Source: CAD feature listing. Evaluate the final solid. Frame: model axes, mm. A direction names the side the tool comes from. Give positions to 0.01 mm unless a question says otherwise; leave off trailing zeros. Order: outer loops, then holes, each group sorted by start corner. A loop starts at its lowest first (then second) coordinate and runs counter-clockwise, first axis right, second up.
1) Section D-D, the plane y = 74.5. Return loops of the section in (x, z) (3 decimals).
2) Section C-C, the plane z = 2.4. Give the number of separate pieces and of enclosed holes in the cut face, plus the area to 3 significant figures.
3) First-contact query: P1, Ø6.5, axis at x = 38.1, y = 12.7, coming from the +Z side (3 decimals); P2, Ø1.6, axis at y = 19.5, z = 2.5, coming from the +X side; P3, Ø1, axis at x = 298.5, z = 2.5, coming from the -Y side; P4, Ø1.6, axis at x = 217, z = 1, coming from the -Y side. Flat tips, straight axial feed; report the tip coordinate or a pass-through.
4) Access query for faces 4 (the face through (125.09, 1.81, 1.61)), 5 (the face through (105.885, 71.607, 1.61)). Directions: +Z, -Z, +X, -X, +Y, -Y. A direction counts if a zero-diameter tool reaches every point of the face in a straight line with its end or side. Return the directions, or none.
5) Draft query along X for faces 1 (the face through (138, 73, 0)), 2 (the face through (32.161, 71.607, 1.61)), 3 (the face through (20, 75.4, 1.6)). Return one class per face: released by +X, released by -X, zero draft, split by the parting line, or undercut.
6) Material intervals for line 1 (X direction, y = 35, z = 1.85); line 2 (X direction, y = 67, z = 1.9); line 3 (Y direction, x = 184, z = 2), sorted ascending.
7) Section A-A, the plane y = 95.5. Return loops of the section in (x, z) (3 decimals).
8) Section B-B, the plane x = 232.5. Return loops of the section in (y, z) (3 decimals), plus the area to 3 significant figures.
```python
from build123d import *

# Parameters (mm, degrees)
SKETCH1_R           = 2.54
SKETCH1_R_2         = 2.159
BOSS_EXTRUDE1_DEPTH = 3.175
FILLET1_R           = 6.35
CUT_EXTRUDE1_DEPTH  = 354.562731103
FILLET2_R           = 3.175
SKETCH3_R           = 2.54
CUT_EXTRUDE2_DEPTH  = 354.562731103
FILLET3_R           = 3.175


with BuildPart() as part:
    # Sketch1 → Boss-Extrude1 (new body)
    with BuildSketch(Plane.XY):
        with BuildLine():
            Line((40.64, 127), (0, 25.4))
            Line((0, 25.4), (0, 0))
            Line((0, 0), (127, 0))
            Line((127, 0), (127, 25.4))
            Line((127, 25.4), (152.4, 88.9))
            Line((152.4, 88.9), (278.011284287, 88.9))
            ThreePointArc((278.011284287, 88.9), (326.39, 107.95), (278.011284287, 127))
            Line((278.011284287, 127), (40.64, 127))
        make_face()
        with Locations((12.7, 12.7)):
            Circle(SKETCH1_R, mode=Mode.SUBTRACT)
        with Locations((38.1, 12.7)):
            Circle(SKETCH1_R, mode=Mode.SUBTRACT)
        with Locations((63.5, 12.7)):
            Circle(SKETCH1_R, mode=Mode.SUBTRACT)
        with Locations((88.9, 12.7)):
            Circle(SKETCH1_R, mode=Mode.SUBTRACT)
        with Locations((114.3, 12.7)):
            Circle(SKETCH1_R, mode=Mode.SUBTRACT)
        with Locations((286.54375, 128.572229928)):
            Circle(SKETCH1_R_2, mode=Mode.SUBTRACT)
        with Locations((310.35625, 128.572229928)):
            Circle(SKETCH1_R_2, mode=Mode.SUBTRACT)
        with Locations((310.35625, 87.327770072)):
            Circle(SKETCH1_R_2, mode=Mode.SUBTRACT)
        with Locations((286.54375, 87.327770072)):
            Circle(SKETCH1_R_2, mode=Mode.SUBTRACT)
        Polygon((302.409468146, 101.092), (294.490531854, 101.092), (290.531063708, 107.95), (294.490531854, 114.808), (302.409468146, 114.808), (306.368936292, 107.95), align=None, mode=Mode.SUBTRACT)
        with Locations((274.6375, 107.95)):
            Circle(SKETCH1_R_2, mode=Mode.SUBTRACT)
        with Locations((322.2625, 107.95)):
            Circle(SKETCH1_R_2, mode=Mode.SUBTRACT)
    extrude(amount=BOSS_EXTRUDE1_DEPTH)

    # Fillet1
    fillet1_edges = [part.edges().sort_by_distance(p)[0] for p in [
        (278.011284287, 88.9, 1.5875),
        (152.4, 88.9, 1.5875),
        (127, 25.4, 1.5875),
        (127, 0, 1.5875),
        (0, 0, 1.5875),
        (0, 25.4, 1.5875),
        (40.64, 127, 1.5875),
        (278.011284287, 127, 1.5875),
    ]]
    fillet(fillet1_edges, radius=FILLET1_R)

    # Sketch2 → Cut-Extrude1 (cut, through all)
    with BuildSketch(Plane.XY.offset(3.175)):
        Polygon((49.23831861, 114.3), (13.67831861, 25.4), (39.597669611, 25.4), (75.157669611, 114.3), align=None)
        Polygon((86.100324499, 114.3), (50.540324499, 25.4), (76.459675501, 25.4), (112.019675501, 114.3), align=None)
        Polygon((122.962330389, 114.3), (87.402330389, 25.4), (113.32168139, 25.4), (148.88168139, 114.3), align=None)
    extrude(amount=-CUT_EXTRUDE1_DEPTH, mode=Mode.SUBTRACT)

    # Fillet2
    fillet2_edges = [part.edges().sort_by_distance(p)[0] for p in [
        (76.459675501, 25.4, 1.5875),
        (50.540324499, 25.4, 1.5875),
        (86.100324499, 114.3, 1.5875),
        (112.019675501, 114.3, 1.5875),
        (148.88168139, 114.3, 1.5875),
        (113.32168139, 25.4, 1.5875),
        (87.402330389, 25.4, 1.5875),
        (122.962330389, 114.3, 1.5875),
        (39.597669611, 25.4, 1.5875),
        (13.67831861, 25.4, 1.5875),
        (49.23831861, 114.3, 1.5875),
        (75.157669611, 114.3, 1.5875),
    ]]
    fillet(fillet2_edges, radius=FILLET2_R)

    # Sketch3 → Cut-Extrude2 (cut, through all)
    with BuildSketch(Plane.XY.offset(3.175)):
        with Locations((45.72, 120.65)):
            Circle(SKETCH3_R)
        with Locations((119.38, 120.65)):
            Circle(SKETCH3_R)
        with Locations((193.04, 120.65)):
            Circle(SKETCH3_R)
        with Locations((266.7, 120.65)):
            Circle(SKETCH3_R)
    extrude(amount=-CUT_EXTRUDE2_DEPTH, mode=Mode.SUBTRACT)

    # Fillet3
    fillet3_edges = [part.edges().sort_by_distance(p)[0] for p in [
        (302.409468146, 101.092, 1.5875),
        (306.368936292, 107.95, 1.5875),
        (302.409468146, 114.808, 1.5875),
        (294.490531854, 114.808, 1.5875),
        (290.531063708, 107.95, 1.5875),
        (294.490531854, 101.092, 1.5875),
    ]]
    fillet(fillet3_edges, radius=FILLET3_R)


solid = part.part
```
From the geometry:
1. outline: (19.64, 0) - (33.318, 0) - (33.318, 3.175) - (19.64, 3.175) - close; (59.238, 0) - (70.18, 0) - (70.18, 3.175) - (59.238, 3.175) - close; (96.1, 0) - (107.042, 0) - (107.042, 3.175) - (96.1, 3.175) - close; (132.962, 0) - (146.64, 0) - (146.64, 3.175) - (132.962, 3.175) - close
2. separate pieces: 1
2. enclosed holes: 19
2. area: 15,600 mm2
3. P1: stops at z = 3.175
3. P2: stops at x = 127
3. P3: stops at y = 80.01
3. P4: stops at y = 88.9
4. face 4: +Z, -Z, +X, -Y
4. face 5: +Z, -Z
5. face 1: zero draft
5. face 2: undercut
5. face 3: released by -X
6. line 1: x = 3.84 to 17.52, 43.44 to 54.38, 80.3 to 91.24, 117.16 to 130.84
6. line 2: x = 16.64 to 30.32, 56.24 to 67.18, 93.1 to 104.04, 129.96 to 143.64
6. line 3: y = 88.9 to 127
7. outline: (28.04, 0) - (41.718, 0) - (41.718, 3.175) - (28.04, 3.175) - close; (67.638, 0) - (78.58, 0) - (78.58, 3.175) - (67.638, 3.175) - close; (104.5, 0) - (115.442, 0) - (115.442, 3.175) - (104.5, 3.175) - close; (141.362, 0) - (323.463, 0) - (323.463, 3.175) - (141.362, 3.175) - close
8. outline: (88.9, 0) - (127, 0) - (127, 3.175) - (88.9, 3.175) - close
8. area: 121 mm2
